Read the model definition and answer for the solid it produces. Units are mm, in the model's axes. A direction names the side the tool comes from. Coordinates: 2 decimals unless noted, no trailing zeros. Loops run counter-clockwise (first coordinate to the right, second up) from the corner with the lowest first, then second, coordinate; pieces in that order, holes last. Notation, with made-up numbers: (56.25, -38) - (86.25, -38) arc R22 ccw to (86.25, -14) - close; hole circle Ø7 at (58.25, 36). An arc over 180 degrees is marked (long way). One line per question, with ' | ' between items. Start each with the question number.
```python
from build123d import *

# Parameters (mm, degrees)
SKETCH2_W           = 76
SKETCH2_H           = 10
SKETCH2_R           = 2.15
BOSS_EXTRUDE1_DEPTH = 25
CUT_EXTRUDE1_DEPTH  = 27
FILLET1_R           = 4


with BuildPart() as part:
    # Sketch2 → Boss-Extrude1 (new body)
    with BuildSketch(Plane(origin=(0, 0, 0), x_dir=(1, 0, 0), z_dir=(0, 1, 0))):
        Rectangle(SKETCH2_W, SKETCH2_H)
        with Locations((-32, 0)):
            Circle(SKETCH2_R, mode=Mode.SUBTRACT)
        Circle(SKETCH2_R, mode=Mode.SUBTRACT)
        with Locations((32, 0)):
            Circle(SKETCH2_R, mode=Mode.SUBTRACT)
    extrude(amount=BOSS_EXTRUDE1_DEPTH)

    # Sketch3 → Cut-Extrude1 (cut)
    with BuildSketch(Plane.XY.offset(5)):
        Polygon((38, 17), (24, 17), (10, 0), (38, 0), align=None)
    extrude(amount=-CUT_EXTRUDE1_DEPTH, mode=Mode.SUBTRACT)

    # Fillet1
    fillet1_edges = [part.edges().sort_by_distance(p)[0] for p in [
        (24, 17, 0),
        (38, 21, 5),
        (-38, 12.5, 5),
        (-38, 12.5, -5),
        (38, 21, -5),
    ]]
    fillet(fillet1_edges, radius=FILLET1_R)


solid = part.part
```
1) The mould has two halves that part along X. Classify faces 3 (the flat face through (16.49, 7.88, 0.07)), 4 (the cylindrical face through (34.05, 20.94, -0.65)), 5 (the cylindrical face through (-36.859, 12.675, 3.797)): released by +X, released by -X, zero draft, split by the parting line, or undercut.
2) The part is cut by section C-C on y = 3.25. Write down the section's boundary in (x, z), and give its area (3 significant figures).
3) Which of the six approach directions +Z, -Z, +X, -X, +Y, -Y give full straight-line access (tool end or side, diameter ignored) to faces 1 (the flat face through (29, 17, 0)), 2 (the flat face through (-0.5, 25, -2.3))?
4) Find the intervals of material crossed by line 1 along X through (y, z) = (19, 0); line 2 along Z through (x, y) = (32, 23.75); line 3 along X through (y, z) = (13.75, 0), in increasing order. Write a range as from..to.
5) The part is cut by section A-A on x = 32. Write down the section's boundary in (y, z), and give its area (3 significant figures).
6) Given pin 1 Ø1 at (x, z) = (15, -0.5) entering from -Y; pin 2 Ø1 at (x, z) = (-1.5, -1.5) entering from +Y; pin 3 Ø3.5 at (x, z) = (-32, 0) entering from +Y; pin 4 Ø3 at (y, z) = (15.5, -3.5) entering from -X, each flat-ended and moving along its own axis, determine where each tip first touches the part or whether it passes through.
7) The part is cut by section D-D on x = 0. Write down the section's boundary in (y, z).
8) The part is cut by section B-B on z = 0. Write down the section's boundary in (x, y).
Answer below:
1) face 3: released by +X | face 4: undercut | face 5: released by -X
2) outline: (-38, -1) arc R4 ccw to (-34, -5) - (12.68, -5) - (12.68, 5) - (-34, 5) arc R4 ccw to (-38, 1) - close; hole circle Ø4.3 at (-32, 0); hole circle Ø4.3 at (0, 0) | area: 471 mm2
3) face 1: +Z, -Z, +X, -Y | face 2: +Z, -Z, +X, -X, +Y
4) line 1: -38..-34.15, -29.85..-2.15, 2.15..29.85, 34.15..38 | line 2: -5..-2.15, 2.15..5 | line 3: -38..-34.15, -29.85..-2.15, 2.15..21.32
5) outline: (17, -5) - (25, -5) - (25, -2.15) - (17, -2.15) - close; (17, 2.15) - (25, 2.15) - (25, 5) - (17, 5) - close | area: 45.6 mm2
6) pin 1: y = 5.46 | pin 2: y = 25 | pin 3: through | pin 4: x = -37.87
7) outline: (0, -5) - (25, -5) - (25, -2.15) - (0, -2.15) - close; (0, 2.15) - (25, 2.15) - (25, 5) - (0, 5) - close
8) outline: (-38, 0) - (-34.15, 0) - (-34.15, 25) - (-38, 25) - close; (-29.85, 0) - (-2.15, 0) - (-2.15, 25) - (-29.85, 25) - close; (2.15, 0) - (10, 0) - (22.8, 15.54) arc R4 cw to (25.89, 17) - (29.85, 17) - (29.85, 25) - (2.15, 25) - close; (34.15, 17) - (38, 17) - (38, 25) - (34.15, 25) - close
